Geometry check sheet. Reference: the model listing, model coordinates, mm. Face numbers are marked on the shaded views. Round coordinates to 2 decimals unless told otherwise and drop trailing zeros. Write each loop counter-clockwise with the first axis right and the second up, starting at its lowest first coordinate (ties: lowest second). Pieces come first, ordered by that corner, then holes.
Item 1: Cross-section at D-D (z = -34.5). Enter the section's corners in (x, y), then the cut area to 3 significant figures.
Item 2: Cross-section at B-B (x = 0). Enter the section's corners in (y, z).
Item 3: Draft check along Z on the marked faces 1, 2 and 3. Enter one of: pulls with the +Z half, pulls with the -Z half, needs draft (parallel to the pull), parting line crosses it, or undercut.
Item 4: Cross-section at A-A (z = 0). Enter the section's corners in (x, y).
Item 5: Cross-section at C-C (x = -21). Enter the section's corners in (y, z), then the cut area to 3 significant figures.
Item 6: Depth check by flat-ended pin: P1, Ø1, axis at y = 6, z = 7.5, coming from the +X side; P2, Ø5, axis at x = 34, z = 8, coming from the -Y side; P3, Ø3, axis at y = 4.5, z = 28, coming from the -X side; P4, Ø1, axis at x = -20, y = 7, coming from the -Z side. Enter the tip coordinate at first touch or a pass-through.
Item 7: Scan lines: probe 1 along X at (y, z) = (1, -27); probe 2 along Z at (x, y) = (-45, 1); probe 3 along X at (y, z) = (2, 6). Record each from-to range of solid material in increasing order.
from build123d import *

# Parameters (mm, degrees)
O_RINGS_PROFILE_W = 2.032
O_RINGS_PROFILE_H = 2.032


with BuildPart() as part:
    # Main Shape Profile → Main Shape (revolve)
    with BuildSketch(Plane.XY, mode=Mode.PRIVATE) as main_shape_sk:
        Polygon((57.15, 0), (57.15, 8.89), (44.45, 8.89), (44.45, 6.35), (6.35, 6.35), (6.35, 8.89), (0, 8.89), (0, 0), align=None)
    revolve(main_shape_sk.sketch.rotate(Axis((0, 0, 0), (0, -1, 0)), 180), axis=Axis((0, 0, 0), (0, -1, 0)))

    # O Rings Profile → O-Rings Cutout (revolve, cut)
    with BuildSketch(Plane.XY, mode=Mode.PRIVATE) as o_rings_cutout_sk:
        with Locations((53.594, 7.874)):
            Rectangle(O_RINGS_PROFILE_W, O_RINGS_PROFILE_H)
        with Locations((53.594, 1.016)):
            Rectangle(O_RINGS_PROFILE_W, O_RINGS_PROFILE_H)
    revolve(o_rings_cutout_sk.sketch.rotate(Axis((0, 0, 0), (0, -1, 0)), 90), axis=Axis((0, 0, 0), (0, -1, 0)), mode=Mode.SUBTRACT)


solid = part.part
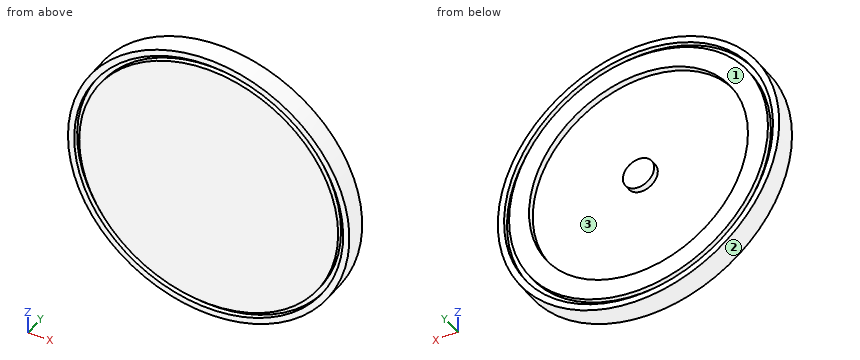
Resolved:
1. outline: (-45.56, 0) - (-42.33, 0) - (-42.33, 2.03) - (-39.68, 2.03) - (-39.68, 0) - (39.68, 0) - (39.68, 2.03) - (42.33, 2.03) - (42.33, 0) - (45.56, 0) - (45.56, 8.89) - (42.33, 8.89) - (42.33, 6.86) - (39.68, 6.86) - (39.68, 8.89) - (28.03, 8.89) - (28.03, 6.35) - (-28.03, 6.35) - (-28.03, 8.89) - (-39.68, 8.89) - (-39.68, 6.86) - (-42.33, 6.86) - (-42.33, 8.89) - (-45.56, 8.89) - close
1. area: 646 mm2
2. outline: (0, -57.15) - (8.89, -57.15) - (8.89, -54.61) - (6.86, -54.61) - (6.86, -52.58) - (8.89, -52.58) - (8.89, -44.45) - (6.35, -44.45) - (6.35, -6.35) - (8.89, -6.35) - (8.89, 6.35) - (6.35, 6.35) - (6.35, 44.45) - (8.89, 44.45) - (8.89, 52.58) - (6.86, 52.58) - (6.86, 54.61) - (8.89, 54.61) - (8.89, 57.15) - (0, 57.15) - (0, 54.61) - (2.03, 54.61) - (2.03, 52.58) - (0, 52.58) - (0, -52.58) - (2.03, -52.58) - (2.03, -54.61) - (0, -54.61) - close
3. face 1: needs draft
3. face 2: parting line crosses it
3. face 3: undercut
4. outline: (-57.15, 0) - (-54.61, 0) - (-54.61, 2.03) - (-52.58, 2.03) - (-52.58, 0) - (52.58, 0) - (52.58, 2.03) - (54.61, 2.03) - (54.61, 0) - (57.15, 0) - (57.15, 8.89) - (54.61, 8.89) - (54.61, 6.86) - (52.58, 6.86) - (52.58, 8.89) - (44.45, 8.89) - (44.45, 6.35) - (6.35, 6.35) - (6.35, 8.89) - (-6.35, 8.89) - (-6.35, 6.35) - (-44.45, 6.35) - (-44.45, 8.89) - (-52.58, 8.89) - (-52.58, 6.86) - (-54.61, 6.86) - (-54.61, 8.89) - (-57.15, 8.89) - close
5. outline: (0, -53.15) - (8.89, -53.15) - (8.89, -50.41) - (6.86, -50.41) - (6.86, -48.2) - (8.89, -48.2) - (8.89, -39.18) - (6.35, -39.18) - (6.35, 39.18) - (8.89, 39.18) - (8.89, 48.2) - (6.86, 48.2) - (6.86, 50.41) - (8.89, 50.41) - (8.89, 53.15) - (0, 53.15) - (0, 50.41) - (2.03, 50.41) - (2.03, 48.2) - (0, 48.2) - (0, -48.2) - (2.03, -48.2) - (2.03, -50.41) - (0, -50.41) - close
5. area: 728 mm2
6. P1: stops at x = 56.72
6. P2: stops at y = 0
6. P3: stops at x = -50.63
6. P4: stops at z = -53.72
7. probe 1: x = -50.37 to -47.47, -45.12 to 45.12, 47.47 to 50.37
7. probe 2: z = -35.23 to -30.94, -27.19 to 27.19, 30.94 to 35.23
7. probe 3: x = -56.83 to -54.28, -52.23 to 52.23, 54.28 to 56.83
